Autodesk Inventor part; units mm, degrees
ref_plane "YZ Plane" through (0, 0, 0) normal (1, 0, 0) x (0, 1, 0)
ref_plane "XZ Plane" through (0, 0, 0) normal (0, 1, 0) x (-1, 0, 0)
ref_plane "XY Plane" through (0, 0, 0) normal (0, 0, 1) x (1, 0, 0)
sketch "Sketch1" plane through (0, 0, 0) normal (0, 1, 0) x (-1, 0, 0)
  line L0 (14.5, 12.75) -> (-14.5, 12.75)
  line L1 (-14.5, 12.75) -> (-14.5, -12.75)
  line L2 (-14.5, -12.75) -> (14.5, -12.75)
  line L3 (14.5, -12.75) -> (14.5, 12.75)
  line L4 (14.5, 12.75) -> (-14.5, -12.75) construction
  line L5 (-14.5, 12.75) -> (14.5, -12.75) construction
  point P0 (0, 0)
  dimension "d0" = 29
  dimension "d1" = 25.5
extrude "Extrusion1" add sketch "Sketch1" along normal mid plane 0.13
sketch "Sketch2" plane through (0, 0.065, 0) normal (0, 1, 0) x (1, 0, 0)
  circle A0 centre (-10.75, 10) radius 1.5
  line L0 (14.5, 12.75) -> (-14.5, 12.75)
  line L1 (-14.5, 12.75) -> (-14.5, -12.75)
  circle A1 centre (10.75, 10) radius 1.5
  circle A2 centre (-10.75, -10) radius 1.5
  circle A3 centre (10.75, -10) radius 1.5
  point P0 (0, 0)
  dimension "d4" = 3
  dimension "d5" = 2.75
  dimension "d6" = 3.75
  dimension "d9" = 21.5
  dimension "d12" = 20
extrude "Extrusion2" cut sketch "Sketch2" against normal through all
sketch "Sketch3" plane through (0, 0.065, 0) normal (0, 1, 0) x (1, 0, 0)
  line L0 (-9.5, 7.25) -> (9.5, 7.25)
  line L1 (9.5, 7.25) -> (9.5, -7.25)
  line L2 (9.5, -7.25) -> (-9.5, -7.25)
  line L3 (-9.5, -7.25) -> (-9.5, 7.25)
  line L4 (-9.5, 7.25) -> (9.5, -7.25) construction
  line L5 (9.5, 7.25) -> (-9.5, -7.25) construction
  point P0 (0, 0)
  dimension "d17" = 19
  dimension "d18" = 14.5
extrude "Extrusion3" cut sketch "Sketch3" against normal through all
properties material "Nylon 6/6"
Source: CAD feature listing. Evaluate the final solid. Frame: model axes, mm. Coordinates: 2 decimals unless noted, no trailing zeros. Write each loop counter-clockwise with the first axis right and the second up, starting at its lowest first coordinate (ties: lowest second). Pieces come first, ordered by that corner, then holes. Notation, with made-up numbers: M 31.5,30.5 L 75.5,30.5 A26 cw 75.5,53.5 Z; hole C 44,-31.5 d2. An arc over 180 degrees is marked long. Answer as a JSON object with one key per item and string values.
1. Cut plane D-D on y = 0. Output: boundary loops of the cut face in (x, z).
Evaluation:
{"outline": "M -14.5,-12.75 L 14.5,-12.75 L 14.5,12.75 L -14.5,12.75 Z; hole C -10.75,-10 d3; hole C -10.75,10 d3; hole M -9.5,-7.25 L 9.5,-7.25 L 9.5,7.25 L -9.5,7.25 Z; hole C 10.75,-10 d3; hole C 10.75,10 d3"}
2. Ray query, L1, parallel to X at y = 0, z = 10; L2, parallel to Z at x = 10.75, y = 0; L3, parallel to Z at x = 2.75, y = 0. Return the intervals inside material, ascending.
Evaluation:
{"L1": "-14.5 to -12.25, -9.25 to 9.25, 12.25 to 14.5", "L2": "-12.75 to -11.5, -8.5 to 8.5, 11.5 to 12.75", "L3": "-12.75 to -7.25, 7.25 to 12.75"}
3. Cut plane A-A on x = -10.75. Output: boundary loops of the cut face in (y, z) (3 decimals).
Evaluation:
{"outline": "M -0.065,-12.75 L 0.065,-12.75 L 0.065,-11.5 L -0.065,-11.5 Z; M -0.065,-8.5 L 0.065,-8.5 L 0.065,8.5 L -0.065,8.5 Z; M -0.065,11.5 L 0.065,11.5 L 0.065,12.75 L -0.065,12.75 Z"}
4. Cut plane B-B on z = -5.5. Output: boundary loops of the cut face in (x, y) (3 decimals).
Evaluation:
{"outline": "M -14.5,-0.065 L -9.5,-0.065 L -9.5,0.065 L -14.5,0.065 Z; M 9.5,-0.065 L 14.5,-0.065 L 14.5,0.065 L 9.5,0.065 Z"}
5. Cut plane C-C on x = 4.5. Output: boundary loops of the cut face in (y, z) (3 decimals), plus the area to 3 significant figures.
Evaluation:
{"outline": "M -0.065,-12.75 L 0.065,-12.75 L 0.065,-7.25 L -0.065,-7.25 Z; M -0.065,7.25 L 0.065,7.25 L 0.065,12.75 L -0.065,12.75 Z", "area": "1.43 mm^2"}
